Verification items for the finished model (mm, model axes). Face numbers are marked on the shaded views. A direction names the side the tool comes from. Coordinates: 2 decimals unless noted, no trailing zeros. Order: outer loops, then holes, each group sorted by start corner. A loop starts at its lowest first (then second) coordinate and runs counter-clockwise, first axis right, second up. Notation, with made-up numbers: M 79,11 L 109,11 A22 cw 109,46 Z; hole C -6.75,-28.5 d8. An arc over 180 degrees is marked long. Use one line per item in the form item = value. Start each with the question number.
```python
from build123d import *

# Parameters (mm, degrees)
SKETCH2_W           = 73.34
SKETCH2_H           = 88.58
BOSS_EXTRUDE1_DEPTH = 3.5
SKETCH1_R           = 1.5875
CUT_EXTRUDE1_DEPTH  = 3.5
BOSS_EXTRUDE2_DEPTH = 63.5
SKETCH4_W           = 73.34
SKETCH4_H           = 88.58
BOSS_EXTRUDE3_DEPTH = 5
SKETCH5_R           = 3
CUT_EXTRUDE2_DEPTH  = 5
SKETCH6_W           = 65.34
SKETCH6_H           = 44.75
BOSS_EXTRUDE4_DEPTH = 15
CUT_EXTRUDE3_DEPTH  = 126.25610564
SKETCH11_R          = 6
CUT_EXTRUDE4_DEPTH  = 131.546436183
CUT_EXTRUDE5_DEPTH  = 11.2


with BuildPart() as part:
    # Sketch2 → Boss-Extrude1 (new body)
    with BuildSketch(Plane(origin=(0, 0, 0), x_dir=(1, 0, 0), z_dir=(0, 1, 0))):
        with Locations((-26.67, 34.29)):
            Rectangle(SKETCH2_W, SKETCH2_H)
    extrude(amount=-BOSS_EXTRUDE1_DEPTH)

    # Sketch1 → Cut-Extrude1 (cut)
    with BuildSketch(Plane(origin=(0, 0, 0), x_dir=(1, 0, 0), z_dir=(0, 1, 0))):
        with Locations(Location((-7.62, 66.04, 0), (0, 0, 270))):
            Circle(SKETCH1_R)
        with Locations(Location((-35.56, 66.04, 0), (0, 0, 270))):
            Circle(SKETCH1_R)
        with Locations(Location((-2.54, 13.97, 0), (0, 0, 270))):
            Circle(SKETCH1_R)
        with Locations(Location((-50.8, 15.24, 0), (0, 0, 270))):
            Circle(SKETCH1_R)
    extrude(amount=-CUT_EXTRUDE1_DEPTH, mode=Mode.SUBTRACT)

    # Sketch3 → Boss-Extrude2 (add)
    with BuildSketch(Plane.XZ.offset(3.5)):
        Polygon((10, -78.58), (-63.34, -78.58), (-63.34, 10), (-55.34, 10), (-55.34, -70.58), (10, -70.58), align=None)
    extrude(amount=BOSS_EXTRUDE2_DEPTH)

    # Sketch4 → Boss-Extrude3 (add)
    with BuildSketch(Plane.XZ.offset(67)):
        with Locations((-26.67, -34.29)):
            Rectangle(SKETCH4_W, SKETCH4_H)
    extrude(amount=BOSS_EXTRUDE3_DEPTH)

    # Sketch5 → Cut-Extrude2 (cut)
    with BuildSketch(Plane.XZ.offset(72)):
        with Locations(Location((-5, -21.59, 0), (0, 0, 270))):
            Circle(SKETCH5_R)
        with Locations(Location((-5, -46.99, 0), (0, 0, 270))):
            Circle(SKETCH5_R)
        with Locations(Location((-40, -21.59, 0), (0, 0, 270))):
            Circle(SKETCH5_R)
        with Locations(Location((-40, -46.99, 0), (0, 0, 270))):
            Circle(SKETCH5_R)
    extrude(amount=-CUT_EXTRUDE2_DEPTH, mode=Mode.SUBTRACT)

    # Sketch6 → Boss-Extrude4 (add)
    with BuildSketch(Plane.XY.offset(-70.58)):
        with Locations((-22.67, -44.625)):
            Rectangle(SKETCH6_W, SKETCH6_H)
    extrude(amount=BOSS_EXTRUDE4_DEPTH)

    # Sketch9 → Cut-Extrude3 (cut, through all)
    with BuildSketch(Plane.XY.offset(-70.58)):
        Polygon((-17.145, -41.747783942), (-17.145, -30.749261314), (-26.67, -25.25), (-36.195, -30.749261314), (-36.195, -41.747783942), (-26.67, -47.247045256), align=None)
    extrude(amount=CUT_EXTRUDE3_DEPTH, mode=Mode.SUBTRACT)

    # Sketch11 → Cut-Extrude4 (cut, through all)
    with BuildSketch(Plane(origin=(0, 0, -78.58), x_dir=(-1, 0, 0), z_dir=(0, 0, -1))):
        with Locations((26.67, -45)):
            Circle(SKETCH11_R)
    extrude(amount=-CUT_EXTRUDE4_DEPTH, mode=Mode.SUBTRACT)

    # Sketch12 → Cut-Extrude5 (cut)
    with BuildSketch(Plane.XY.offset(-70.58)):
        Polygon((-17.145, -39.500738686), (-26.67, -34.001477372), (-36.195, -39.500738686), (-36.195, -50.499261314), (-26.67, -55.998522628), (-17.145, -50.499261314), align=None)
    extrude(amount=CUT_EXTRUDE5_DEPTH, mode=Mode.SUBTRACT)


solid = part.part
```
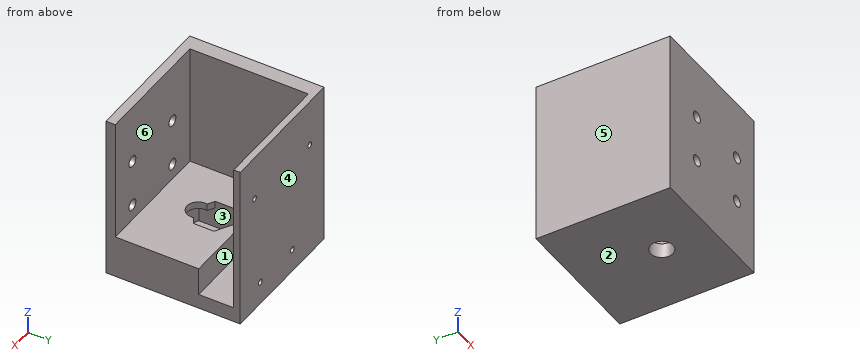
1. Tool access check on the marked faces 1, 2 and 3. Record the directions out of +Z, -Z, +X, -X, +Y, -Y that give a thin tool (end or side, any length) a straight path to the whole face; none if there is none.
2. Cross-section at C-C on x = -40. Enter the section's corners in (y, z), and give its area (3 significant figures).
3. Release check for a two-part mould opening along Y. For the marked faces 4, 5 and 6 record: pulls with the +Y half, pulls with the -Y half, needs draft (parallel to the pull), parting line crosses it, or undercut.
4. Cross-section at B-B on x = -50.8. Enter the section's corners in (y, z).
5. Material ranges on line 1 along X through (y, z) = (-68.45, -21.59); line 2 along X through (y, z) = (-1, -66); line 3 along Y through (x, z) = (-47, -15), recorded low to high.
6. Cross-section at A-A on z = -66.04. Give the number of separate pieces and of enclosed holes in the cut face, and give its area (3 significant figures).
7. Depth check by flat-ended pin: P1, Ø19, axis at y = -25.5, z = -45.5, coming from the +X side; P2, Ø19.5, axis at x = -25.5, z = -20, coming from the +Y side; P3, Ø15, axis at x = -22.5, y = -46.5, coming from the +Z side. Enter the tip coordinate at first touch or a pass-through.
8. Cross-section at D-D on y = -53. Enter the section's corners in (x, z).
Final values:
q1.face_1 = +Z, +X
q1.face_2 = -Z, +X, -X, +Y, -Y
q1.face_3 = none
q2.outline = M -72,-78.58 L 0,-78.58 L 0,10 L -3.5,10 L -3.5,-70.58 L -22.25,-70.58 L -22.25,-55.58 L -67,-55.58 L -67,-49.99 L -72,-49.99 Z; M -72,-43.99 L -67,-43.99 L -67,-24.59 L -72,-24.59 Z; M -72,-18.59 L -67,-18.59 L -67,10 L -72,10 Z
q2.area = 1,870 mm2
q3.face_4 = pulls with the +Y half
q3.face_5 = needs draft
q3.face_6 = undercut
q4.outline = M -72,-78.58 L 0,-78.58 L 0,-16.83 L -3.5,-16.83 L -3.5,-70.58 L -22.25,-70.58 L -22.25,-55.58 L -67,-55.58 L -67,10 L -72,10 Z; M -3.5,-13.65 L 0,-13.65 L 0,10 L -3.5,10 Z
q5.line_1 = -63.34 to -43, -37 to -8, -2 to 10
q5.line_2 = -63.34 to -37.15, -33.97 to -9.21, -6.03 to 10
q5.line_3 = -72 to -67, -3.5 to 0
q6.separate_pieces = 3
q6.enclosed_holes = 1
q6.area = 3,550 mm2
q7.P1 = -55.34
q7.P2 = 0
q7.P3 = -55.58
q8.outline = M -63.34,-78.58 L 10,-78.58 L 10,-55.58 L -55.34,-55.58 L -55.34,10 L -63.34,10 Z; hole M -31.86,-70.58 L -21.48,-70.58 L -21.48,-59.38 L -31.86,-59.38 Z
